Part model, mm, in its own coordinate system. Round coordinates to 2 decimals unless told otherwise and drop trailing zeros. Loops run counter-clockwise (first coordinate to the right, second up) from the corner with the lowest first, then second, coordinate; pieces in that order, holes last.
(1) Probe probe 1 along X at (y, z) = (-13.5, 1.9); probe 2 along X at (y, z) = (-22.5, 2.5); probe 3 along Y at (x, z) = (-69.85, 1.8). List the from-to ranges inside material, lowest first.
(2) Cut at A-A on z = 2.3. List the corners of the cut face in (x, y), then the cut area to 3 significant figures.
(3) Mould opens along X. For faces 1 (the face through (56.2, -17, 1.6)), 2 (the face through (88.01, -30.46, 1.57)), 3 (the face through (-1, 38.1, 2)) say: +X half, -X half, draft (parallel to the pull), parting line (faces both ways), or undercut.
(4) Cut at B-B on x = -72. List the corners of the cut face in (y, z) (1 decimal), then the cut area to 3 significant figures.
(5) Cut at C-C on y = -16. List the corners of the cut face in (x, z) (3 decimals), then the cut area to 3 significant figures.
from build123d import *

# Parameters (mm, degrees)
SKETCH1_R           = 14.3129
BOSS_EXTRUDE1_DEPTH = 3.175


with BuildPart() as part:
    # Sketch1 → Boss-Extrude1 (new body)
    with BuildSketch(Plane.XY):
        with BuildLine():
            Line((69.85, -38.1), (-69.85, -38.1))
            ThreePointArc((-69.85, -38.1), (-87.810512242, -30.660512242), (-95.25, -12.7))
            Line((-95.25, -12.7), (-95.25, 38.1))
            Line((-95.25, 38.1), (95.25, 38.1))
            Line((95.25, 38.1), (95.25, -12.7))
            ThreePointArc((95.25, -12.7), (87.810512242, -30.660512242), (69.85, -38.1))
        make_face()
        with Locations((-69.85, -12.7)):
            Circle(SKETCH1_R, mode=Mode.SUBTRACT)
        with Locations(Location((69.85, -12.7, 0), (0, 0, 180))):
            Circle(SKETCH1_R, mode=Mode.SUBTRACT)
    extrude(amount=BOSS_EXTRUDE1_DEPTH)


solid = part.part
Final values:
1. probe 1: x = -95.24 to -84.14, -55.56 to 55.56, 84.14 to 95.24
1. probe 2: x = -93.28 to -80.28, -59.42 to 59.42, 80.28 to 93.28
1. probe 3: y = -38.1 to -27.01, 1.61 to 38.1
2. outline: (-95.25, -12.7) arc R25.4 ccw to (-69.85, -38.1) - (69.85, -38.1) arc R25.4 ccw to (95.25, -12.7) - (95.25, 38.1) - (-95.25, 38.1) - close; hole circle Ø28.63 at (-69.85, -12.7); hole circle Ø28.63 at (69.85, -12.7)
2. area: 13,000 mm2
3. face 1: undercut
3. face 2: +X half
3. face 3: draft
4. outline: (-38, 0) - (-26.9, 0) - (-26.9, 3.2) - (-38, 3.2) - close; (1.5, 0) - (38.1, 0) - (38.1, 3.2) - (1.5, 3.2) - close
4. area: 152 mm2
5. outline: (-95.035, 0) - (-83.777, 0) - (-83.777, 3.175) - (-95.035, 3.175) - close; (-55.923, 0) - (55.923, 0) - (55.923, 3.175) - (-55.923, 3.175) - close; (83.777, 0) - (95.035, 0) - (95.035, 3.175) - (83.777, 3.175) - close
5. area: 427 mm2
